The model under review builds one solid part; all positions refer to its coordinate system, in mm. Face numbers are marked on the shaded views. Give positions to 0.01 mm unless a question says otherwise; leave off trailing zeros. Order: outer loops, then holes, each group sorted by start corner. A loop starts at its lowest first (then second) coordinate and runs counter-clockwise, first axis right, second up. Notation, with made-up numbers: M 43.5,-31.75 L 76.5,-31.75 A33 cw 76.5,4.25 Z; hole C 45,36.5 d3. An arc over 180 degrees is marked long. One line per question, with ' | ' between items. Start each with the question number.
1. The part is to be moulded in two halves that separate along Z. For the marked faces 1, 2 and 3, say which applies: +Z half, -Z half, draft (parallel to the pull), parting line (faces both ways), or undercut.
2. Insertion check: P1, Ø3, axis at x = -20.5, y = 39, coming from the -Z side; P2, Ø3, axis at y = 19.5, z = 12.5, coming from the +X side; P3, Ø1.5, axis at x = 0, y = 6, coming from the -Z side. Each pin has a flat end and moves straight along its axis. Give the tip position at first contact, or say it passes through.
3. We need section A-A on y = 24. Write out the cut boundary in (x, z), then the cut area to 3 significant figures.
4. We need section B-B on y = 29. Write out the cut boundary in (x, z).
5. Wall thickness on L1, parallel to X at y = 2.75, z = 0; L2, parallel to X at y = 32.5, z = -2.5; L3, parallel to Z at x = -8, y = 16: over which ranges is each line inside the solid? List them lowest first.
```python
from build123d import *

# Parameters (mm, degrees)
SKETCH1_R           = 13.25
SKETCH1_R_2         = 10.25
BOSS_EXTRUDE1_DEPTH = 10
FILLET1_R           = 10


with BuildPart() as part:
    # Sketch1 → Boss-Extrude1 (new body)
    with BuildSketch(Plane(origin=(0, 0, 0), x_dir=(1, 0, 0), z_dir=(0, 1, 0))):
        with Locations(Location((0, 0, 0), (0, 0, 270))):
            Circle(SKETCH1_R)
        with Locations(Location((0, 0, 0), (0, 0, 270))):
            Circle(SKETCH1_R_2, mode=Mode.SUBTRACT)
    extrude(amount=BOSS_EXTRUDE1_DEPTH)

    # Sketch2 → Revolve1 (revolve)
    with BuildSketch(Plane.XY, mode=Mode.PRIVATE) as revolve1_sk:
        Polygon((-13.25, 10), (-33.25, 44.641016151), (-30.25, 44.641016151), (-10.25, 10), align=None)
    revolve(revolve1_sk.sketch.rotate(Axis((0, 0, 0), (0, 1, 0)), 270), axis=Axis((0, 0, 0), (0, 1, 0)))

    # Fillet1
    fillet1_edges = [part.edges().sort_by_distance(p)[0] for p in [
        (-10.25, 10, 0),
    ]]
    fillet(fillet1_edges, radius=FILLET1_R)


solid = part.part
```
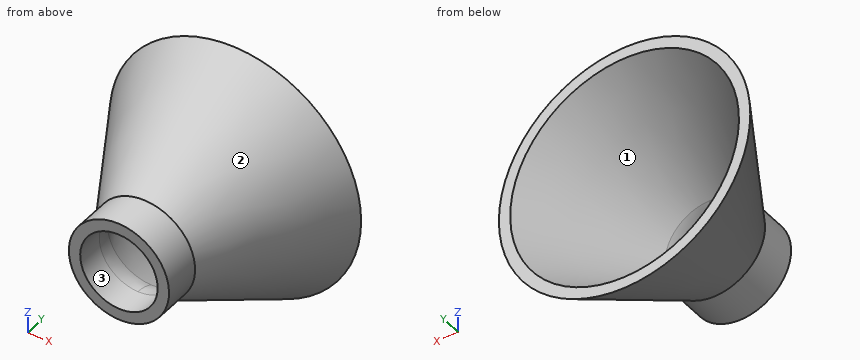
Entries:
1) face 1: undercut | face 2: parting line | face 3: undercut
2) P1: stops at z = -23.64 | P2: stops at x = 15.6 | P3: stops at z = -13.25
3) outline: C 0,0 d42.67; hole C 0,0 d36.67 | area: 374 mm^2
4) outline: C 0,0 d48.44; hole C 0,0 d42.44
5) L1: x = -13.25 to -10.25, 10.25 to 13.25 | L2: x = -26.12 to -23.11, 23.11 to 26.12 | L3: z = -14.68 to -11.14, 11.14 to 14.68
